Source: three-view drawing plus pictorial views. Frame: mm from the lowest corner of the part. A direction names the side the tool comes from. Give positions to 0.01 mm unless a question says otherwise; leave off trailing zeros. Write each loop counter-clockwise with the first axis right and the second up, starting at its lowest first coordinate (ties: lowest second). Pieces come first, ordered by that corner, then holes. Notation, with made-up numbers: (80.5, 3) -> (105.5, 3) arc R20 ccw to (105.5, 7) -> close; hole circle Ø2 at (39, 51.25). An arc over 180 degrees is marked (long way). Answer in a Markdown table with one row per item. Add a question column.
Item 1: Draft query along X for the marked faces 1, 2 and 3. Return one class per face: +X half, -X half, draft (parallel to the pull), parting line (faces both ways), or undercut.
Item 2: Section query B-B on z = 86. Output: boundary loops of the cut face in (x, y).
Item 3: Section query C-C on x = 217.5. Output: boundary loops of the cut face in (y, z), plus the area to 3 significant figures.
Item 4: Material intervals for probe 1 along X at (y, z) = (87, 22); probe 2 along Y at (x, z) = (133.5, 84); probe 3 along Z at (x, y) = (127, 24), sorted ascending. Write a range as from..to.
Item 5: Section query A-A on z = 11. Output: boundary loops of the cut face in (x, y).
Item 6: Access query for the marked faces 4 and 5. Directions: +Z, -Z, +X, -X, +Y, -Y. A direction counts if a zero-diameter tool reaches every point of the face in a straight line with its end or side. Return the directions, or none.
Item 7: Section query D-D on y = 25. Output: boundary loops of the cut face in (x, z).
Item 8: First-contact query: P1, Ø1.5, axis at x = 247, y = 52.5, coming from the +Z side; P2, Ø1, axis at y = 43.5, z = 39, coming from the -X side; P3, Ø4, axis at x = 2, y = 37, coming from the +Z side; P4, Ø10, axis at x = 157, y = 101.5, coming from the -Z side. Flat tips, straight axial feed; report the tip coordinate or a pass-through.
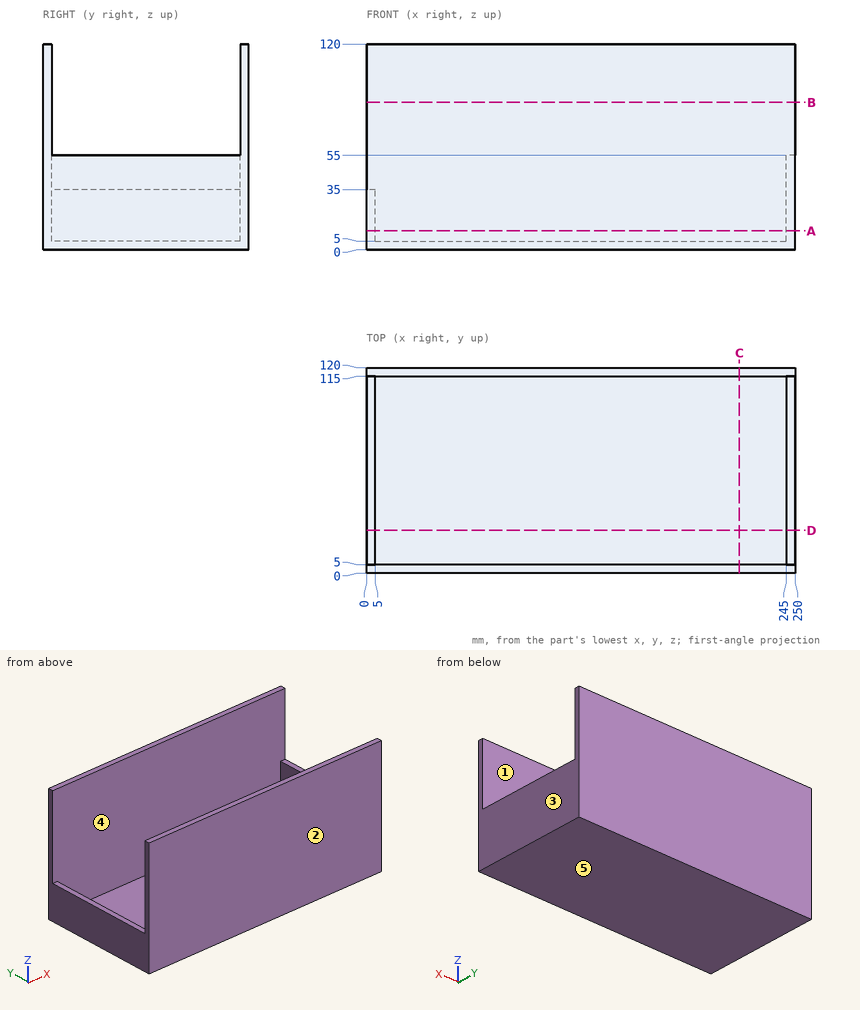
Findings below:
| question | item | result |
|---|---|---|
| 1 | face 1 | undercut |
| 1 | face 2 | draft |
| 1 | face 3 | +X half |
| 2 | outline | (0, 0) -> (250, 0) -> (250, 5) -> (0, 5) -> close; (0, 115) -> (250, 115) -> (250, 120) -> (0, 120) -> close |
| 3 | outline | (0, 0) -> (120, 0) -> (120, 120) -> (115, 120) -> (115, 5) -> (5, 5) -> (5, 120) -> (0, 120) -> close |
| 3 | area | 1,750 mm^2 |
| 4 | probe 1 | x = 0..5, 245..250 |
| 4 | probe 2 | y = 0..5, 115..120 |
| 4 | probe 3 | z = 0..5 |
| 5 | outline | (0, 0) -> (250, 0) -> (250, 120) -> (0, 120) -> close; hole (5, 5) -> (245, 5) -> (245, 115) -> (5, 115) -> close |
| 6 | face 4 | +Z |
| 6 | face 5 | -Z, +X, -X, +Y, -Y |
| 7 | outline | (0, 0) -> (250, 0) -> (250, 55) -> (245, 55) -> (245, 5) -> (5, 5) -> (5, 35) -> (0, 35) -> close |
| 8 | P1 | stops at z = 55 |
| 8 | P2 | stops at x = 245 |
| 8 | P3 | stops at z = 35 |
| 8 | P4 | stops at z = 0 |
